The model under review builds one solid part; all positions refer to its coordinate system, in mm. Face numbers are marked on the shaded views. A direction names the side the tool comes from. Round coordinates to 2 decimals unless told otherwise and drop trailing zeros. Write each loop counter-clockwise with the first axis right and the second up, starting at its lowest first coordinate (ties: lowest second). Pieces come first, ordered by that corner, then holes. Notation, with made-up numbers: (-3.75, 58.25) -> (41.25, 58.25) arc R12 cw to (41.25, 67.25) -> close; hole circle Ø8 at (84.25, 23). An arc over 180 degrees is marked (long way). Answer as a JSON object with one key per item and string values. Group by question number.
1) Mouldability with a two-part tool opening along Y and no side actions: class the marked faces 4, 5 and 6 as pulls with the +Y half, pulls with the -Y half, needs draft (parallel to the pull), parting line crosses it, or undercut.
2) Machinability: for the marked faces 1, 2 and 3, which of the approach directions +Z, -Z, +X, -X, +Y, -Y give a long, thin tool a straight path to every point of the face, cutting with its end or side? Answer none if there is none.
3) Insertion check: pin 1 Ø6 at (x, z) = (5, -26.5) entering from +Y; pin 2 Ø4 at (x, y) = (16.5, 150.5) entering from -Z; pin 3 Ø7 at (x, y) = (15.5, -10) entering from +Z. Each pin has a flat end and moves straight along its axis. Give the tip position at first contact, or say it passes through.
4) We need section D-D, the plane y = 90. Write out the cut boundary in (x, z), then the cut area to 3 significant figures.
5) We need section A-A, the plane z = 0. Write out the cut boundary in (x, y), then the cut area to 3 significant figures.
6) To check wall thickness, follow probe 1 along Y at (x, z) = (24, -59.5); probe 2 along Y at (x, z) = (16, -50.5); probe 3 along Z at (x, y) = (21.75, 70.5). State the ranges of each line that lie inside material, in increasing order. Write a range as [from, to].
7) We need section B-B, the plane x = 13.5. Write out the cut boundary in (y, z) (1 decimal), then the cut area to 3 significant figures.
8) We need section C-C, the plane z = -17. Write out the cut boundary in (x, y).
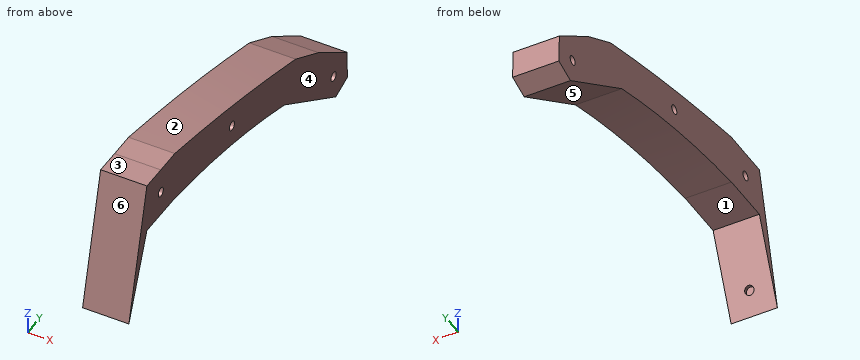
Autodesk Fusion 360 part; units mm, degrees
sketch "Sketch1" plane through (0, 0, 0) normal (1, 0, 0) x (0, 1, 0)
  circle A0 centre (0, 0) radius 2.6
  circle A1 centre (175.9096, -53.4375) radius 2.6
  line L0 (137.2781, -14.356) -> (160.424, -26.9456)
  line L1 (160.424, -26.9456) -> (189.4776, -47.6848)
  line L2 (189.4776, -47.6848) -> (189.9997, -63.9991)
  line L3 (189.9997, -63.9991) -> (178.1831, -67.9555)
  line L4 (178.1831, -67.9555) -> (125.9198, -35.3622)
  circle A2 centre (72.465, -10.0775) radius 2.6
  line L5 (-14.2, 14.2002) -> (-32.5668, -60.5772)
  line L6 (0, 14.2002) -> (14.2, 14.3859)
  line L7 (0, 14.2002) -> (-14.2, 14.2002)
  line L8 (0, -14.2002) -> (14.2, -14.2002)
  line L9 (0, -14.2002) -> (-14.2, -14.2002)
  line L10 (-14.2, -14.2002) -> (-32.5668, -60.5772)
  arc A3 (137.2781, -14.356) -> (14.2, 14.3859) centre (-186.9778, -1124.9865) ccw
  arc A4 (125.9198, -35.3622) -> (14.2, -14.2002) centre (-22.4488, -513.1589) ccw
  dimension "d1" = 5.2
  dimension "d7" = 5.2
  dimension "d37" = 5.2
  dimension "d40" = 77
extrude "Extrude1" add sketch "Sketch1" along normal mid plane 52
sketch "Sketch2" plane through (0, -16.6815, 4.0973) normal (0, -0.9711, 0.2385) x (1, 0, 0)
  line L0 (26, -66.5968) -> (26, 10.4032)
extrude "Extrude2" cut 1 faces at (-26, 27.9887, 2.1627) along direction (1, 0, 0) blind 26
sketch "Sketch3" plane through (0, -16.6815, 4.0973) normal (0, -0.9711, 0.2385) x (1, 0, 0)
  line L0 (0, 10.4032) -> (0, -66.5968)
  line L1 (0, -66.5968) -> (26, -66.5968)
  line L2 (26, -66.5968) -> (26, 10.4032)
  line L3 (26, 10.4032) -> (0, 10.4032)
  circle A0 centre (13, -53.0968) radius 2.6
  dimension "d53" = 5.2
extrude "Extrude3" cut sketch "Sketch3" against normal blind 5 contours A0
Here are the results:
{
 "1": {"face 4": "needs draft", "face 5": "undercut", "face 6": "pulls with the -Y half"},
 "2": {"face 1": "-Z, +X, -X", "face 2": "+Z, +X, -X, +Y", "face 3": "+Z, +X, -X, -Y"},
 "3": {"pin 1": "stops at y = 164", "pin 2": "stops at z = -51.94", "pin 3": "stops at z = 14.2"},
 "4": {"outline": "(0, -25.66) -> (26, -25.66) -> (26, -1.63) -> (0, -1.63) -> close", "area": "625 mm^2"},
 "5": {"outline": "(0, -17.69) -> (26, -17.69) -> (26, -2.6) -> (0, -2.6) -> close; (0, 2.6) -> (26, 2.6) -> (26, 83.29) -> (0, 83.29) -> close", "area": "2,490 mm^2"},
 "6": {"probe 1": "y = [-32.3, -32.14], [164.62, 189.86]", "probe 2": "y = [-30.09, -28.58], [150.19, 189.57]", "probe 3": "z = [-21.57, -11.78], [-8.37, 3]"},
 "7": {"outline": "(-32.6, -60.6) -> (-28.5, -50.3) -> (-30, -49.9) -> (-28.7, -45) -> (-26.6, -45.5) -> (-14.2, -14.2) -> (14.2, -14.2) arc R500.3 cw to (125.9, -35.4) -> (178.2, -68) -> (190, -64) -> (189.5, -47.7) -> (160.4, -26.9) -> (137.3, -14.4) arc R1157 ccw to (14.2, 14.4) -> (0, 14.2) -> (-14.2, 14.2) -> close; hole circle Ø5.2 at (0, 0); hole circle Ø5.2 at (72.5, -10.1); hole circle Ø5.2 at (175.9, -53.4)", "area": "5,550 mm^2"},
 "8": {"outline": "(0, -21.86) -> (26, -21.86) -> (26, -15.31) -> (0, -15.31) -> close; (0, 41.81) -> (26, 41.81) -> (26, 142.14) -> (0, 142.14) -> close"}
}
